For this review, take the finished solid that the model builds, in its own axes (mm). A direction names the side the tool comes from. Coordinates: 2 decimals unless noted, no trailing zeros. Write each loop counter-clockwise with the first axis right and the second up, starting at its lowest first coordinate (ties: lowest second). Pieces come first, ordered by that corner, then holes.
1) For faces 4 (the face through (13.1, 16.9, -2.7)), 5 (the face through (-9.075, 26, -3)), 6 (the face through (4.15, 11, -4)), 7 (the face through (6, 8, -3)), 8 (the face through (16.63, -2.85, -2.79)), list the 3-axis set-ups (+Z, -Z, +X, -X, +Y, -Y) from which the entire face can be reached by the end or side of a thin tool; tool diameter is ignored.
2) We need section C-C on y = 0.5. Write out the cut boundary in (x, z) (3 decimals).
3) We need section D-D on x = 10.8. Write out the cut boundary in (y, z).
4) We need section A-A on y = 4.25. Write out the cut boundary in (x, z) (3 decimals), then the cut area to 3 significant figures.
5) Mouldability with a two-part tool opening along Y and no side actions: class faces 1 (the face through (0, 23.6, -4)), 2 (the face through (-17, 4, -3)), 3 (the face through (-9.136, 24.235, -2.788)) as pulls with the +Y half, pulls with the -Y half, needs draft (parallel to the pull), parting line crosses it, or undercut.
6) We need section B-B on z = -3.85. Give the number of separate pieces and of enclosed holes in the cut face, then the cut area to 3 significant figures.
7) Insertion check: P1, Ø1.1, axis at y = 24.5, z = -1, coming from the -X side; P2, Ø3, axis at x = 8, y = 14.5, coming from the +Z side; P3, Ø0.8, axis at y = 13.5, z = -3.5, coming from the -X side; P4, Ø2.5, axis at x = 10.8, y = 4.25, coming from the +Z side. Each pin has a flat end and moves straight along its axis. Give the tip position at first contact, or say it passes through.
8) To check wall thickness, follow line 1 along X through (y, z) = (7, -1.9) (3 decimals); line 2 along Y through (x, z) = (1, -3.55) (3 decimals); line 3 along Y through (x, z) = (-5, -0.25) (3 decimals). State the ranges of each line that lie inside material, in increasing order.
Autodesk Inventor part; units mm, degrees
ref_plane "YZ Plane" through (0, 0, 0) normal (1, 0, 0) x (0, 1, 0)
ref_plane "XZ Plane" through (0, 0, 0) normal (0, 1, 0) x (-1, 0, 0)
ref_plane "XY Plane" through (0, 0, 0) normal (0, 0, 1) x (1, 0, 0)
sketch "Sketch1" plane through (0, 0, 0) normal (0, 0, 1) x (1, 0, 0)
  line L0 (-5, -2.5) -> (5, -2.5) construction
  line L1 (5, -2.5) -> (12.675, 0) construction
  line L2 (-5, -2.5) -> (-12.675, 0)
  line L3 (12.675, 0) -> (-12.675, 0) construction
  line L4 (12.675, 0) -> (12.675, 8.7) construction
  line L5 (-12.675, 0) -> (-12.675, 8.7)
  line L6 (-12.675, 8.7) -> (-4.75, 23.1)
  line L7 (-4.75, 23.1) -> (-4.75, 25.1)
  line L8 (-4.75, 25.1) -> (4.75, 25.1) construction
  line L9 (4.75, 25.1) -> (4.75, 23.1) construction
  line L10 (4.75, 23.1) -> (12.675, 8.7) construction
  line L11 (0, -8.44) -> (0, 31.04)
  line L12 (0, 25.1) -> (0, -2.5)
  circle A0 centre (-10.8, 4.25) radius 1.25
  line L13 (-10.8, 4.25) -> (0, 4.25) construction
  line L14 (-4.75, 25.1) -> (0, 25.1)
  line L15 (-5, -2.5) -> (0, -2.5)
  line L16 (-5.05, 23.1771) -> (-12.975, 8.7771)
  line L17 (-12.975, 8.7771) -> (-12.975, -0.2178)
  line L18 (-12.975, -0.2178) -> (-5.0476, -2.8)
  line L19 (-5.0476, -2.8) -> (0.3, -2.8) construction
  line L20 (0.3, -2.8) -> (0.3, 25.4) construction
  line L21 (0.3, 25.4) -> (-5.05, 25.4) construction
  line L22 (-5.05, 25.4) -> (-5.05, 23.1771)
  line L23 (0, -2.5) -> (0, -2.8)
  line L24 (0, 25.1) -> (0, 25.4)
  line L25 (0, -2.8) -> (-5.0476, -2.8)
  line L26 (0, 25.4) -> (-5.05, 25.4)
  point P0 (0, 0)
  point P1 (0, 0)
  dimension "d0" = 10
  dimension "d1" = 25.35
  dimension "d2" = 2.5
  dimension "d3" = 8.7
  dimension "d4" = 27.6
  dimension "d6" = 2
  dimension "d7" = 9.5
  dimension "d42" = 2.5
  dimension "d43" = 10.8
  dimension "d44" = 6.75
  dimension "d53" = 0.3
sketch "Sketch8" plane through (0, 0, 0) normal (0, 0, 1) x (1, 0, 0)
  line L0 (-20, 30) -> (20, 30)
  line L1 (20, 30) -> (20, -10)
  line L2 (20, -10) -> (-20, -10)
  line L3 (-20, -10) -> (-20, 30)
  point P0 (0, 0)
  point P1 (0, -10)
  dimension "d45" = 40
  dimension "d46" = 10
extrude "MainBlock" add sketch "Sketch8" against normal blind 5.5
extrude "CartridgeCutout" cut sketch "Sketch1" against normal blind 3
sketch "Sketch10" plane through (-10.8, 4.25, 0) normal (0, 0, 1) x (1, 0, 0)
  circle A0 centre (0, 0) radius 1.25
  circle A1 centre (0, 0) radius 1.45
  point P0 (10.8, -4.25)
  dimension "d56" = 0.2
extrude "PinHole" cut sketch "Sketch10" against normal through all contours A0 | A1
mirror "Mirror3" about plane through (0, 25.4, 0) normal (-1, 0, 0) of "CartridgeCutout", "PinHole"
sketch "Sketch12" plane through (0, 0, -3) normal (0, 0, 1) x (1, 0, 0)
  circle A0 centre (10.8, 4.25) radius 1.45
  circle A1 centre (-10.8, 4.25) radius 1.45
  line L0 (5.05, 25.4) -> (-5.05, 25.4)
  line L1 (-5.05, 23.1771) -> (-5.05, 25.4)
  line L2 (-12.975, 8.7771) -> (-5.05, 23.1771)
  line L3 (-12.975, -0.2178) -> (-12.975, 8.7771)
  line L4 (-5.0476, -2.8) -> (-12.975, -0.2178)
  line L5 (5.0476, -2.8) -> (-5.0476, -2.8)
  line L6 (5.0476, -2.8) -> (12.975, -0.2178)
  line L7 (12.975, -0.2178) -> (12.975, 8.7771)
  line L8 (12.975, 8.7771) -> (5.05, 23.1771)
  line L9 (5.05, 23.1771) -> (5.05, 25.4)
  line L10 (-4.15, 23.6) -> (4.15, 23.6)
  line L11 (4.15, 23.6) -> (4.15, -1.4)
  line L12 (4.15, -1.4) -> (-4.15, -1.4)
  line L13 (-4.15, -1.4) -> (-4.15, 23.6)
  point P0 (0, 0)
  point P1 (0, -1.4)
  dimension "d59" = 8.3
  dimension "d60" = 25
  dimension "d61" = 1.4
extrude "Extrusion12" cut sketch "Sketch12" against normal through all contours L10 L11 L12 L13
sketch "Sketch13" plane through (0, 0, 0) normal (0, 0, 1) x (1, 0, 0)
  line L0 (-5.05, 25.4) -> (5.05, 25.4)
  line L1 (5.05, 25.4) -> (5.05, 23.1771)
  line L2 (5.05, 23.1771) -> (12.975, 8.7771)
  line L3 (12.975, 8.7771) -> (12.975, -0.2178)
  line L4 (12.975, -0.2178) -> (5.0476, -2.8)
  line L5 (5.0476, -2.8) -> (-5.0476, -2.8)
  line L6 (-5.0476, -2.8) -> (-12.975, -0.2178)
  line L7 (-12.975, -0.2178) -> (-12.975, 8.7771)
  line L8 (-12.975, 8.7771) -> (-5.05, 23.1771)
  line L9 (-5.05, 23.1771) -> (-5.05, 25.4)
  line L10 (-20, 30) -> (20, 30)
  line L11 (-20, -10) -> (-20, 30)
  line L12 (20, -10) -> (-20, -10)
  line L13 (20, 30) -> (20, -10)
  line L14 (-17, 9.8115) -> (-17, -3.1399)
  line L15 (-17, -3.1399) -> (-5.6866, -6.825)
  line L16 (-5.6866, -6.825) -> (5.6866, -6.825)
  line L17 (5.6866, -6.825) -> (17, -3.1399)
  line L18 (17, -3.1399) -> (17, 9.8115)
  line L19 (17, 9.8115) -> (9.075, 24.2115)
  line L20 (9.075, 24.2115) -> (9.075, 29.425)
  line L21 (9.075, 29.425) -> (-9.075, 29.425)
  line L22 (-9.075, 29.425) -> (-9.075, 24.2115)
  line L23 (-9.075, 24.2115) -> (-17, 9.8115)
  point P0 (0, 0)
  dimension "d65" = 4.025
extrude "Extrusion13" cut sketch "Sketch13" against normal through all contours L10 L13 L12 L11
fillet "Fillet2" radius 2 10 edges at (-9.075, 29.425, -2.75) (9.075, 29.425, -2.75) (9.075, 24.2115, -2.75) (17, 9.8115, -2.75) (17, -3.1399, -2.75) (5.6866, -6.825, -2.75) (-5.6866, -6.825, -2.75) (-17, -3.1399, -2.75) (-9.075, 24.2115, -2.75) (-17, 9.8115, -2.75)
properties part number "InkjetHolderV2"
Result:
1. face 4: +Z, -Z, +X, +Y
1. face 5: +Z, -Z, -X, +Y
1. face 6: +Z, -Z
1. face 7: +Z
1. face 8: +Z, -Z, +X, -Y
2. outline: (-17, -5.5) - (-4.15, -5.5) - (-4.15, -3) - (-12.975, -3) - (-12.975, 0) - (-17, 0) - close; (4.15, -5.5) - (17, -5.5) - (17, 0) - (12.975, 0) - (12.975, -3) - (4.15, -3) - close
3. outline: (-5.16, -5.5) - (2.8, -5.5) - (2.8, -3) - (-0.93, -3) - (-0.93, 0) - (-5.16, 0) - close; (5.7, -5.5) - (21.08, -5.5) - (21.08, 0) - (12.73, 0) - (12.73, -3) - (5.7, -3) - close
4. outline: (-17, -5.5) - (-12.25, -5.5) - (-12.25, -3) - (-12.975, -3) - (-12.975, 0) - (-17, 0) - close; (-9.35, -5.5) - (-4.15, -5.5) - (-4.15, -3) - (-9.35, -3) - close; (4.15, -5.5) - (9.35, -5.5) - (9.35, -3) - (4.15, -3) - close; (12.25, -5.5) - (17, -5.5) - (17, 0) - (12.975, 0) - (12.975, -3) - (12.25, -3) - close
4. area: 73.9 mm2
5. face 1: undercut
5. face 2: needs draft
5. face 3: pulls with the +Y half
6. separate pieces: 1
6. enclosed holes: 3
6. area: 771 mm2
7. P1: stops at x = -9.23
7. P2: stops at z = -3
7. P3: stops at x = -15.19
7. P4: passes through
8. line 1: x = -17 to -12.975, 12.975 to 17
8. line 2: y = -6.825 to -1.4, 23.6 to 29.425
8. line 3: y = -6.825 to -2.8, 25.4 to 29.425
